```python
from build123d import *

# Parameters (mm, degrees)
DODANIE_WYCI_GNI_CIE1_DEPTH = 7


with BuildPart() as part:
    # Szkic1 → Obrót1 (revolve)
    with BuildSketch(Plane.XY):
        Polygon((0, 0), (-23.1, 0), (-23.1, 21.15), (-16.8, 25.8), (-16.8, 36.3), (-8, 36.3), (-8, 22.3), (0, 22.3), align=None)
    revolve(axis=Axis((0, 22.3, 0), (0, -1, 0)))

    # Szkic2 → Dodanie-wyciągnięcie1 (add)
    with BuildSketch(Plane(origin=(0, 36.3, 0), x_dir=(1, 0, 0), z_dir=(0, 1, 0))):
        with BuildLine():
            Line((-7.729655239, 21.23705323), (-5.745938408, 15.786836029))
            ThreePointArc((-5.745938408, 15.786836029), (0, 16.8), (5.745938408, 15.786836029))
            Line((5.745938408, 15.786836029), (7.729655239, 21.23705323))
            ThreePointArc((7.729655239, 21.23705323), (0, 22.6), (-7.729655239, 21.23705323))
        make_face()
        with BuildLine():
            ThreePointArc((15.786836029, 5.745938408), (16.8, 0), (15.786836029, -5.745938408))
            Line((15.786836029, -5.745938408), (21.23705323, -7.729655239))
            ThreePointArc((21.23705323, -7.729655239), (22.6, 0), (21.23705323, 7.729655239))
            Line((21.23705323, 7.729655239), (15.786836029, 5.745938408))
        make_face()
        with BuildLine():
            ThreePointArc((5.745938408, -15.786836029), (0, -16.8), (-5.745938408, -15.786836029))
            Line((-5.745938408, -15.786836029), (-7.729655239, -21.23705323))
            ThreePointArc((-7.729655239, -21.23705323), (0, -22.6), (7.729655239, -21.23705323))
            Line((7.729655239, -21.23705323), (5.745938408, -15.786836029))
        make_face()
        with BuildLine():
            ThreePointArc((-15.786836029, -5.745938408), (-16.8, 0), (-15.786836029, 5.745938408))
            Line((-15.786836029, 5.745938408), (-21.23705323, 7.729655239))
            ThreePointArc((-21.23705323, 7.729655239), (-22.6, 0), (-21.23705323, -7.729655239))
            Line((-21.23705323, -7.729655239), (-15.786836029, -5.745938408))
        make_face()
    extrude(amount=-DODANIE_WYCI_GNI_CIE1_DEPTH)


solid = part.part
```
Design review of the part built by this model. Coordinates are the model's own, in mm. A direction names the side the tool comes from. Give positions to 0.01 mm unless a question says otherwise; leave off trailing zeros. Order: outer loops, then holes, each group sorted by start corner. A loop starts at its lowest first (then second) coordinate and runs counter-clockwise, first axis right, second up. Notation, with made-up numbers: M 65,66 L 104,66 A26 cw 104,88 Z; hole C 88.25,-18 d9. An arc over 180 degrees is marked long. One line per question, with ' | ' between items. Start each with the question number.
Q1. For pin 1 Ø2 at (x, y) = (9, 14) entering from -Z; pin 2 Ø6 at (x, z) = (10.5, -17.5) entering from +Y; pin 3 Ø12 at (x, y) = (15, 4) entering from +Z, all flat-tipped, find the tip position at first contact; note any pin that passes through.
Q2. We need section A-A (y = 34.5). Write out the cut boundary in (x, z).
Q3. Machinability: for faces 1 (the face through (0, 22.3, 0)), 2 (the face through (-0.1, 32.8, 22.6)), 3 (the face through (-6.724, 32.849, 18.474)), which of the approach directions +Z, -Z, +X, -X, +Y, -Y give a long, thin tool a straight path to every point of the face, cutting with its end or side? Answer none if there is none.
Q4. We need section C-C (x = 0). Write out the cut boundary in (y, z), plus the area to 3 significant figures.
Q5. We need section D-D (y = 8.5). Write out the cut boundary in (x, z), plus the area to 3 significant figures.
Q6. The part is to be moulded in two halves that separate along X. For faces 4 (the face through (-18.474, 32.849, -6.724)), 5 (the face through (22.6, 32.8, 0.1)), 6 (the face through (1.73, 29.2, 7.81)), 7 (the face through (0.1, 32.8, -22.6)), say which applies: +X half, -X half, draft (parallel to the pull), parting line (faces both ways), or undercut.
Q7. For L1, parallel to X at y = 28, z = 0; L2, parallel to Z at x = 0, y = 25, list the stretches that pass through material, from the lowest coordinate up. Write a range as [from, to].
Q8. We need section B-B (z = 0). Write out the cut boundary in (x, y), plus the area to 3 significant figures.
Returned:
1) pin 1: z = -21.67 | pin 2: y = 25.35 | pin 3: z = 21.27
2) outline: M -21.24,-7.73 L -15.79,-5.75 A16.8 ccw -5.75,-15.79 L -7.73,-21.24 A22.6 ccw 7.73,-21.24 L 5.75,-15.79 A16.8 ccw 15.79,-5.75 L 21.24,-7.73 A22.6 ccw 21.24,7.73 L 15.79,5.75 A16.8 ccw 5.75,15.79 L 7.73,21.24 A22.6 ccw -7.73,21.24 L -5.75,15.79 A16.8 ccw -15.79,5.75 L -21.24,7.73 A22.6 ccw Z; hole C 0,0 d16
3) face 1: +Y | face 2: +Z, +Y | face 3: -X, +Y
4) outline: M 0,-23.1 L 21.15,-23.1 L 25.8,-16.8 L 29.3,-16.8 L 29.3,-22.6 L 36.3,-22.6 L 36.3,-8 L 22.3,-8 L 22.3,8 L 36.3,8 L 36.3,22.6 L 29.3,22.6 L 29.3,16.8 L 25.8,16.8 L 21.15,23.1 L 0,23.1 Z | area: 1,370 mm2
5) outline: C 0,0 d46.2 | area: 1,680 mm2
6) face 4: undercut | face 5: +X half | face 6: undercut | face 7: parting line
7) L1: [-16.8, -8], [8, 16.8] | L2: [-17.88, -8], [8, 17.88]
8) outline: M -23.1,0 L 23.1,0 L 23.1,21.15 L 16.8,25.8 L 16.8,29.3 L 22.6,29.3 L 22.6,36.3 L 8,36.3 L 8,22.3 L -8,22.3 L -8,36.3 L -22.6,36.3 L -22.6,29.3 L -16.8,29.3 L -16.8,25.8 L -23.1,21.15 Z | area: 1,370 mm2
